For this review, take the finished solid that the model builds, in its own axes (mm). Face numbers are marked on the shaded views. A direction names the side the tool comes from. Round coordinates to 2 decimals unless told otherwise and drop trailing zeros. Write each loop counter-clockwise with the first axis right and the second up, starting at its lowest first coordinate (ties: lowest second). Pieces come first, ordered by that corner, then holes.
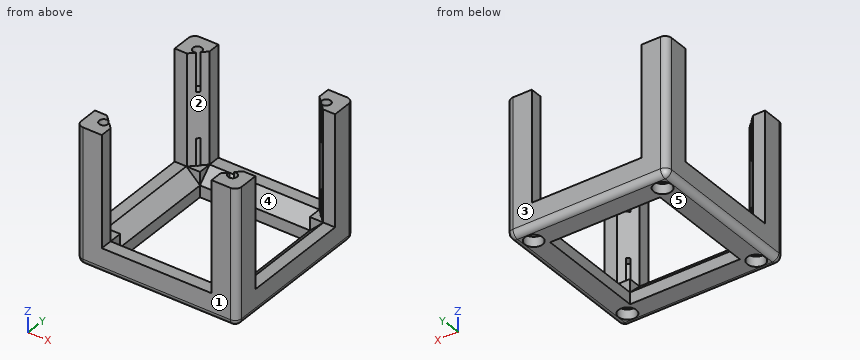
Autodesk Inventor part; units mm, degrees
ref_plane "YZ Plane" through (0, 0, 0) normal (1, 0, 0) x (0, 1, 0)
ref_plane "XZ Plane" through (0, 0, 0) normal (0, 1, 0) x (-1, 0, 0)
ref_plane "XY Plane" through (0, 0, 0) normal (0, 0, 1) x (1, 0, 0)
sketch "Sketch1" plane through (0, 0, 0) normal (0, 0, 1) x (1, 0, 0)
  line L0 (-24.9, 24.9) -> (24.9, 24.9)
  line L1 (24.9, 24.9) -> (24.9, -24.9)
  line L2 (24.9, -24.9) -> (-24.9, -24.9)
  line L3 (-24.9, -24.9) -> (-24.9, 24.9)
  line L4 (-24.9, 24.9) -> (24.9, -24.9) construction
  line L5 (24.9, 24.9) -> (-24.9, -24.9) construction
  line L6 (17.05, 17.05) -> (-17.05, 17.05)
  line L7 (-17.05, 17.05) -> (-17.05, -17.05)
  line L8 (-17.05, -17.05) -> (17.05, -17.05)
  line L9 (17.05, -17.05) -> (17.05, 17.05)
  point P0 (0, 0)
  dimension "d0" = 49.8
  dimension "d1" = 49.8
  dimension "d2" = 7.85
extrude "Extrusion1" add sketch "Sketch1" along normal blind 7.7
sketch "Sketch2" plane through (0, 0, 7.7) normal (0, 0, 1) x (1, 0, 0)
  line L0 (17.05, 17.05) -> (17.05, -17.05)
  line L1 (17.05, -17.05) -> (-17.05, -17.05)
  line L2 (-17.05, -17.05) -> (-17.05, 17.05)
  line L3 (-17.05, 17.05) -> (17.05, 17.05)
  line L4 (24.9, 24.9) -> (-24.9, 24.9)
  line L5 (-24.9, 24.9) -> (-24.9, -24.9)
  line L6 (-24.9, -24.9) -> (24.9, -24.9)
  line L7 (24.9, -24.9) -> (24.9, 24.9)
  line L8 (17.05, -17.05) -> (24.9, -17.05)
  line L9 (24.9, -17.05) -> (24.9, -24.9)
  line L10 (24.9, -24.9) -> (17.05, -24.9)
  line L11 (17.05, -24.9) -> (17.05, -17.05)
  line L12 (17.05, 17.05) -> (-17.05, 17.05)
  line L13 (24.9, 24.9) -> (17.05, 24.9)
  line L14 (17.05, 24.9) -> (17.05, 17.05)
  line L15 (17.05, 17.05) -> (24.9, 17.05)
  line L16 (24.9, 17.05) -> (24.9, 24.9)
  line L17 (-24.9, -24.9) -> (-17.05, -24.9)
  line L18 (-17.05, -24.9) -> (-17.05, -17.05)
  line L19 (-17.05, -17.05) -> (-24.9, -17.05)
  line L20 (-24.9, -17.05) -> (-24.9, -24.9)
  line L21 (-24.9, 24.9) -> (-17.05, 24.9)
  line L22 (-17.05, 24.9) -> (-17.05, 17.05)
  line L23 (-17.05, 17.05) -> (-24.9, 17.05)
  line L24 (-24.9, 17.05) -> (-24.9, 24.9)
  point P0 (0, 0)
extrude "Extrusion2" add sketch "Sketch2" along normal blind 34.4 contours L14 L4 L7 L15 | L8 L7 L6 L11 | L23 L5 L4 L22 | L18 L6 L5 L19
sketch "Sketch3" plane through (0, 0, 0) normal (0, 0, -1) x (-1, 0, 0)
  line L0 (24.9, -24.9) -> (24.9, 24.9) construction
  line L1 (24.9, 24.9) -> (-24.9, 24.9) construction
  line L2 (-24.9, -24.9) -> (24.9, -24.9) construction
  line L3 (-24.9, 24.9) -> (-24.9, -24.9) construction
  point P0 (20, 20)
  point P1 (20, -20)
  point P2 (-20, -20)
  point P3 (-20, 20)
  dimension "d_1" = 4.9
  dimension "d96" = 4.9
  dimension "d97" = 4.9
  dimension "d98" = 4.9
  dimension "d99" = 4.9
  dimension "d100" = 4.9
  dimension "d101" = 4.9
  dimension "d102" = 4.9
hole "Hole1" at (-20, 20, 0) at (-20, -20, 0) at (20, -20, 0) at (20, 20, 0) direction (0, 0, 1) diameter 2.8 depth 16 counterbore diameter 5.5 counterbore depth 3.1
fillet "Fillet1" radius 2 8 edges at (24.9, 24.9, 21.05) (24.9, -24.9, 21.05) (-24.9, -24.9, 21.05) (-24.9, 24.9, 21.05) (-24.9, 0, 0) (0, -24.9, 0) (24.9, 0, 0) (0, 24.9, 0)
sketch "Sketch6" plane through (0, 0, 42.1) normal (0, 0, 1) x (1, 0, 0)
  arc A0 (-22.9, 24.9) -> (-24.9, 22.9) centre (-22.9, 22.9) ccw
  line L0 (-24.9, 22.9) -> (-24.9, 17.05)
  line L1 (-24.9, 17.05) -> (-17.05, 17.05)
  line L2 (-17.05, 17.05) -> (-17.05, 24.9)
  line L3 (-17.05, 24.9) -> (-22.9, 24.9)
  arc A1 (24.9, 22.9) -> (22.9, 24.9) centre (22.9, 22.9) ccw
  line L4 (22.9, 24.9) -> (17.05, 24.9)
  line L5 (17.05, 24.9) -> (17.05, 17.05)
  line L6 (17.05, 17.05) -> (24.9, 17.05)
  line L7 (24.9, 17.05) -> (24.9, 22.9)
  arc A2 (22.9, -24.9) -> (24.9, -22.9) centre (22.9, -22.9) ccw
  line L8 (24.9, -22.9) -> (24.9, -17.05)
  line L9 (24.9, -17.05) -> (17.05, -17.05)
  line L10 (17.05, -17.05) -> (17.05, -24.9)
  line L11 (17.05, -24.9) -> (22.9, -24.9)
  arc A3 (-24.9, -22.9) -> (-22.9, -24.9) centre (-22.9, -22.9) ccw
  line L12 (-22.9, -24.9) -> (-17.05, -24.9)
  line L13 (-17.05, -24.9) -> (-17.05, -17.05)
  line L14 (-17.05, -17.05) -> (-24.9, -17.05)
  line L15 (-24.9, -17.05) -> (-24.9, -22.9)
  line L16 (0, 38.1838) -> (54, 38.1838) construction
  line L17 (21.1338, 17.05) -> (17.05, 21.1338)
  line L18 (17.05, 24.9) -> (17.05, 17.05)
  line L19 (17.05, 21.1338) -> (17.05, 17.05)
  line L20 (17.05, 17.05) -> (21.1338, 17.05)
  line L21 (-17.05, 24.9) -> (-17.05, 17.05)
  line L22 (-17.05, 17.05) -> (-17.05, 21.1338)
  line L23 (-17.05, 21.1338) -> (-21.1338, 17.05)
  line L24 (-17.05, 21.1338) -> (-11.2747, 21.1338) construction
  line L25 (-17.05, -17.05) -> (-17.05, 17.05)
  line L26 (-21.1338, 17.05) -> (-17.05, 17.05)
  line L27 (-17.05, 17.05) -> (-21.1338, 17.05)
  line L28 (17.05, -17.05) -> (17.05, -24.9)
  line L29 (17.05, -17.05) -> (21.1338, -17.05)
  line L30 (24.9, -17.05) -> (17.05, -17.05)
  line L31 (21.1338, -17.05) -> (17.05, -21.1338)
  line L32 (17.05, -17.05) -> (17.05, -21.1338)
  line L33 (-17.05, -17.05) -> (-21.1338, -17.05)
  line L34 (-17.05, -17.05) -> (-17.05, -24.9)
  line L35 (-17.05, -17.05) -> (-17.05, -21.1338)
  line L36 (-21.1338, -17.05) -> (-17.05, -21.1338)
  line L37 (22.9, 22.9) -> (24.9, 22.9) construction
  line L38 (-22.9, -22.9) -> (22.9, 22.9) construction
  line L39 (-22.9, -22.9) -> (22.9, -22.9) construction
  line L40 (22.9, 22.9) -> (-22.9, 22.9) construction
  line L41 (22.9, -22.9) -> (-22.9, 22.9) construction
  dimension "d111" = 0
  dimension "d120" = 54
  dimension "d121" = 54
extrude "Extrusion3" cut sketch "Sketch6" against normal up to surface (34.4 mm away) contours L13 L36 L14 | L2 L1 L23 | L6 L5 L17 | L10 L9 L31
sketch "Sketch7" plane through (-24.9, 17.05, 7.7) normal (0, -1, 0) x (1, 0, 0)
  line L0 (41.95, 0) -> (49.95, 0) construction
  line L1 (41.95, -7.7) -> (41.95, 0) construction
  line L2 (7.85, -7.7) -> (7.85, 0) construction
  line L3 (-0.15, 0) -> (7.85, 0) construction
  line L4 (41.9235, 33.7204) -> (41.95, 0) construction
  line L5 (7.85, 0) -> (7.8764, 33.5861) construction
  line L6 (41.95, 0) -> (7.85, 0) construction
  circle A0 centre (24.9, 17.0366) radius 17.0366 construction
  line L7 (24.9, 55.2203) -> (-13.2838, 17.0366) construction
  line L8 (-13.2838, 17.0366) -> (24.9, -21.1472) construction
  line L9 (24.9, -21.1472) -> (63.0838, 17.0366) construction
  line L10 (63.0838, 17.0366) -> (24.9, 55.2203) construction
  line L11 (24.9, 55.2203) -> (24.9, -21.1472) construction
  line L12 (-13.2838, 17.0366) -> (63.0838, 17.0366) construction
  line L13 (24.9, 55.2203) -> (78.9, 55.2203) construction
  line L14 (46.1838, 0) -> (41.95, 0)
  line L15 (46.1838, 0) -> (41.95, -4.0972)
  line L16 (41.95, 0) -> (41.9235, 33.7204)
  line L17 (41.95, 0) -> (41.95, -4.0972)
  line L18 (46.1838, 0) -> (41.95, 0)
  line L19 (41.95, 0) -> (46.1838, 0)
  line L20 (7.85, 0) -> (3.6162, 0)
  line L21 (3.6162, 0) -> (7.85, -4.0972)
  line L22 (7.85, -4.0972) -> (7.85, 0)
  line L23 (24.9, -36.4773) -> (24.9, 70.8333)
  point P0 (44.386, 0)
  point P1 (43.5978, 0)
  point P2 (24.9, 17.0366)
  dimension "d37" = 54
  dimension "d38" = 135
  dimension "d39" = 54
extrude "Extrusion4" cut sketch "Sketch7" along normal up to surface (34.1 mm away)
sketch "Sketch8" plane through (17.05, -24.9, 7.7) normal (-1, 0, 0) x (0, 0, 1)
  line L0 (-4.0838, 41.95) -> (0, 41.95) construction
  line L1 (-4.0838, 7.85) -> (0.1503, 7.85) construction
  line L2 (0.1503, 7.85) -> (0.1503, 3.6159) construction
  line L3 (-4.0838, 7.85) -> (0.1503, 3.6159)
  line L4 (0.1503, 3.6159) -> (0.1503, 7.85)
  line L5 (0.1503, 7.85) -> (-4.0838, 7.85)
  line L6 (-4.0838, 41.95) -> (0, 46.0338)
  line L7 (-4.0838, 41.95) -> (1.6916, 41.95) construction
  line L8 (0.1503, 7.85) -> (0, 41.95)
  line L9 (0, 46.0338) -> (0, 41.95)
  line L10 (0, 41.95) -> (-4.0838, 41.95)
  line L11 (-6, 2) -> (-6, 47.8)
  line L12 (55.2338, 24.9) -> (17.05, 63.0838) construction
  line L13 (17.05, 63.0838) -> (-21.1338, 24.9) construction
  line L14 (-21.1338, 24.9) -> (17.05, -13.2838) construction
  line L15 (17.05, -13.2838) -> (55.2338, 24.9) construction
  line L16 (55.2338, 24.9) -> (-21.1338, 24.9) construction
  line L17 (17.05, 63.0838) -> (17.05, -13.2838) construction
  line L18 (-36.2573, 24.9) -> (70.6573, 24.9) construction
  line L19 (17.05, -28.5573) -> (17.05, 78.3573) construction
  line L20 (0, 41.95) -> (0, 43.5978) construction
  line L21 (0, 7.85) -> (-4.0972, 7.85) construction
  line L22 (-4.0972, 41.95) -> (-4.0972, 7.85) construction
  line L23 (0, 41.95) -> (-4.0972, 41.95) construction
  line L24 (0, 7.85) -> (0, 41.95) construction
  point P0 (-2.4341, 8)
  point P1 (0, 5.414)
  point P2 (17.05, 24.9)
  point P3 (17.05, 24.9)
  point P4 (17.05, 24.9)
  dimension "d122" = 54
  dimension "d123" = 54
extrude "Extrusion5" cut sketch "Sketch8" along normal up to surface (34.1 mm away)
sketch "Sketch9" plane through (0, 0, 42.1) normal (0, 0, 1) x (1, 0, 0)
  arc A0 (19.486, 18.6978) -> (18.6978, 19.486) centre (20, 20) ccw
  arc A1 (18.6978, -19.486) -> (19.486, -18.6978) centre (20, -20) ccw
  arc A2 (-19.486, -18.6978) -> (-18.6978, -19.486) centre (-20, -20) ccw
  arc A3 (-18.6978, 19.486) -> (-19.486, 18.6978) centre (-20, 20) ccw
hole "Hole2" at (20, 20, 42.1) at (-20, 20, 42.1) at (20, -20, 42.1) at (-20, -20, 42.1) direction (0, 0, -1) diameter 2.8 depth 12
sketch "Sketch15" plane through (0, 0, 0) normal (0, 0, -1) x (-1, 0, 0)
  line L0 (-17.05, -17.05) -> (-17.05, 17.05) construction
  line L1 (-17.05, 17.05) -> (17.05, 17.05) construction
  line L2 (17.05, 17.05) -> (17.05, -17.05) construction
  line L3 (17.05, -17.05) -> (-17.05, -17.05) construction
  circle A0 centre (-20, 20) radius 2.75 construction
  circle A1 centre (20, -20) radius 2.75 construction
  circle A2 centre (20, 20) radius 2.75 construction
  circle A3 centre (-20, -20) radius 2.75 construction
  line L4 (-22.9, 22.9) -> (22.9, 22.9) construction
  line L5 (-22.9, -22.9) -> (-22.9, 22.9) construction
  line L6 (22.9, -22.9) -> (-22.9, -22.9) construction
  line L7 (22.9, 22.9) -> (22.9, -22.9) construction
  line L8 (17.05, 21.1338) -> (-17.05, 21.1338) construction
  point P0 (0, 0)
  point P1 (-20.8, -14.5)
  point P2 (-14.5, -20.8)
  point P3 (14.5, -20.8)
  point P4 (20.8, -14.5)
  point P5 (20.8, 14.5)
  point P6 (14.5, 20.8)
  point P7 (-14.5, 20.8)
  point P8 (-20.8, 14.5)
hole "Hole8" [suppressed]
ref_plane "Arbeitsebene2" through (24.9, 0, 0) normal (-0.7071, 0, -0.7071) x (0, 1, 0)
ref_plane "Arbeitsebene3" through (0, -17.05, 7.7) normal (1, 0, 0) x (0, 0, -1)
ref_plane "Work Plane4" through (-17.05, 0, 7.7) normal (0, 1, 0) x (1, 0, 0)
equation "\"d1\" = d0"
equation "\"d121\" = d120"
properties part number "10_Cube_1x1_v3"
(1) Mouldability with a two-part tool opening along Y and no side actions: class the marked faces 3, 4 and 5 as pulls with the +Y half, pulls with the -Y half, needs draft (parallel to the pull), parting line crosses it, or undercut.
Geometry check:
face 3: pulls with the +Y half
face 4: undercut
face 5: needs draft
(2) We need section A-A, the plane z = 23.5. Give the boundary of the cut face in (x, y), and give its area (3 significant figures).
Geometry check:
outline: (-24.9, -22.9) arc R2 ccw to (-22.9, -24.9) - (-17.05, -24.9) - (-17.05, -21.13) - (-21.13, -17.05) - (-24.9, -17.05) - close; (-24.9, 17.05) - (-21.13, 17.05) - (-17.05, 21.13) - (-17.05, 24.9) - (-22.9, 24.9) arc R2 ccw to (-24.9, 22.9) - close; (17.05, -24.9) - (22.9, -24.9) arc R2 ccw to (24.9, -22.9) - (24.9, -17.05) - (21.13, -17.05) - (17.05, -21.13) - close; (17.05, 21.13) - (21.13, 17.05) - (24.9, 17.05) - (24.9, 22.9) arc R2 ccw to (22.9, 24.9) - (17.05, 24.9) - close
area: 210 mm2
(3) We need section B-B, the plane y = -11. Give the boundary of the cut face in (x, z).
Geometry check:
outline: (-24.9, 2) arc R2 ccw to (-22.9, 0) - (-17.05, 0) - (-17.05, 3.6) - (-21.28, 7.7) - (-24.9, 7.7) - close; (17.05, 0) - (22.9, 0) arc R2 ccw to (24.9, 2) - (24.9, 7.7) - (21.28, 7.7) - (17.05, 3.6) - close
(4) For pin 1 Ø1.9 at (x, y) = (7.5, -23) entering from +Z; pin 2 Ø0.8 at (x, y) = (-20, -19.5) entering from -Z; pin 3 Ø3.5 at (x, y) = (-20, 20) entering from -Z, all flat-tipped, find the tip position at first contact; note any pin that passes through.
Geometry check:
pin 1: stops at z = 7.7
pin 2: stops at z = 16
pin 3: stops at z = 3.1
(5) We need section D-D, the plane z = 14. State how many separate pieces and enclosed holes the cut face has, and give its area (3 significant figures).
Geometry check:
separate pieces: 4
enclosed holes: 0
area: 185 mm2
(6) For line 1 along X through (y, z) = (20, 11.75); line 2 along X through (y, z) = (14, 3), list the stretches that pass through material, from the lowest coordinate up.
Geometry check:
line 1: x = -24.9 to -21.4, -18.6 to -18.18, 18.18 to 18.6, 21.4 to 24.9
line 2: x = -24.9 to -17.05, 17.05 to 24.9
(7) For the marked faces 1 and 2, list the 3-axis set-ups (+Z, -Z, +X, -X, +Y, -Y) from which the entire face can be reached by the end or side of a thin tool; tool diameter is ignored.
Geometry check:
face 1: +Z, -Z, +X, -X, -Y
face 2: +Z
(8) We need section C-C, the plane x = -4. Give the boundary of the cut face in (y, z), and give its area (3 significant figures).
Geometry check:
outline: (-24.9, 2) arc R2 ccw to (-22.9, 0) - (-17.05, 0) - (-17.05, 3.62) - (-21.13, 7.7) - (-24.9, 7.7) - close; (17.05, 0) - (22.9, 0) arc R2 ccw to (24.9, 2) - (24.9, 7.7) - (21.13, 7.7) - (17.05, 3.62) - close
area: 102 mm2
